from build123d import *

# Parameters (mm, degrees)
SKETCH1_W           = 80
SKETCH1_H           = 80
BOSS_EXTRUDE1_DEPTH = 14.5
FILLET1_R           = 2
FILLET2_R           = 4
SKETCH2_R           = 5.75
CUT_EXTRUDE1_DEPTH  = 2
SKETCH3_R           = 1.5
CUT_EXTRUDE2_DEPTH  = 12
SKETCH6_R           = 6
CUT_EXTRUDE3_DEPTH  = 2


with BuildPart() as part:
    # Sketch1 → Boss-Extrude1 (new, symmetric)
    with BuildSketch(Plane.XY):
        Rectangle(SKETCH1_W, SKETCH1_H)
    extrude(amount=BOSS_EXTRUDE1_DEPTH, both=True)

    # Fillet1
    fillet1_edges = [part.edges().sort_by_distance(p)[0] for p in [
        (-40, 0, 14.5),
        (0, -40, 14.5),
        (40, 0, 14.5),
        (0, 40, 14.5),
    ]]
    fillet(fillet1_edges, radius=FILLET1_R)

    # Fillet2
    # the kernel refuses this fillet: 4 mm, written as the material it takes off along each edge
    with BuildSketch(Plane(origin=(-36, -36, 14.5), x_dir=(-1, 0, 0), z_dir=(0, 1, 0))) as fillet2_piece_1:
        with BuildLine():
            CenterArc((2, -2), 2, 0, 90)
            Line((4, -2), (4, 0))
            Line((4, 0), (2, 0))
        make_face()
    revolve(axis=Axis((-36, -36, 14.5), (0, 0, 1)), revolution_arc=90, mode=Mode.SUBTRACT)
    with BuildSketch(Plane(origin=(-36, 36, 14.5), x_dir=(0, 1, 0), z_dir=(1, 0, 0))) as fillet2_piece_2:
        with BuildLine():
            CenterArc((2, -2), 2, 0, 90)
            Line((4, -2), (4, 0))
            Line((4, 0), (2, 0))
        make_face()
    revolve(axis=Axis((-36, 36, 14.5), (0, 0, 1)), revolution_arc=90, mode=Mode.SUBTRACT)
    with BuildSketch(Plane(origin=(36, -36, 14.5), x_dir=(0, -1, 0), z_dir=(-1, 0, 0))) as fillet2_piece_3:
        with BuildLine():
            CenterArc((2, -2), 2, 0, 90)
            Line((4, -2), (4, 0))
            Line((4, 0), (2, 0))
        make_face()
    revolve(axis=Axis((36, -36, 14.5), (0, 0, 1)), revolution_arc=90, mode=Mode.SUBTRACT)
    with BuildSketch(Plane(origin=(36, 36, 14.5), x_dir=(1, 0, 0), z_dir=(0, -1, 0))) as fillet2_piece_4:
        with BuildLine():
            CenterArc((2, -2), 2, 0, 90)
            Line((4, -2), (4, 0))
            Line((4, 0), (2, 0))
        make_face()
    revolve(axis=Axis((36, 36, 14.5), (0, 0, 1)), revolution_arc=90, mode=Mode.SUBTRACT)
    with BuildSketch(Plane(origin=(40, 40, 14.5), x_dir=(-1, 0, 0), z_dir=(0, 0, -1)), Plane(origin=(40, -40, 14.5), x_dir=(0, 1, 0), z_dir=(0, 0, -1)), Plane(origin=(-40, -40, -24.5), x_dir=(0, 1, 0), z_dir=(0, 0, 1)), Plane(origin=(-40, 40, -24.5), x_dir=(1, 0, 0), z_dir=(0, 0, 1))) as fillet2_piece_5:
        with BuildLine():
            CenterArc((FILLET2_R, -FILLET2_R), FILLET2_R, 90, 90)
            Line((0, -FILLET2_R), (0, 0))
            Line((0, 0), (FILLET2_R, 0))
        make_face()
    extrude(amount=39, mode=Mode.SUBTRACT)

    # Sketch2 → Cut-Extrude1 (cut)
    with BuildSketch(Plane.XY.offset(14.5)):
        with Locations((-27.6, 30.4)):
            Circle(SKETCH2_R)
        with Locations((-11.8, 30.4)):
            Circle(SKETCH2_R)
        with Locations((7.5, 30.4)):
            Circle(SKETCH2_R)
        with Locations((23.3, 30.4)):
            Circle(SKETCH2_R)
    extrude(amount=-CUT_EXTRUDE1_DEPTH, mode=Mode.SUBTRACT)

    # Sketch3 → Cut-Extrude2 (cut)
    with BuildSketch(Plane.XY.offset(14.5)):
        with Locations((-33.45, 21.95)):
            Circle(SKETCH3_R)
        with Locations((33.55, 21.95)):
            Circle(SKETCH3_R)
        with Locations((-33.45, -33.05)):
            Circle(SKETCH3_R)
        with Locations((33.55, -33.05)):
            Circle(SKETCH3_R)
    extrude(amount=-CUT_EXTRUDE2_DEPTH, mode=Mode.SUBTRACT)

    # Sketch6 → Cut-Extrude3 (cut)
    with BuildSketch(Plane.XY.offset(14.5)):
        with Locations((28.6, -16.4)):
            Circle(SKETCH6_R)
    extrude(amount=-CUT_EXTRUDE3_DEPTH, mode=Mode.SUBTRACT)


solid = part.part
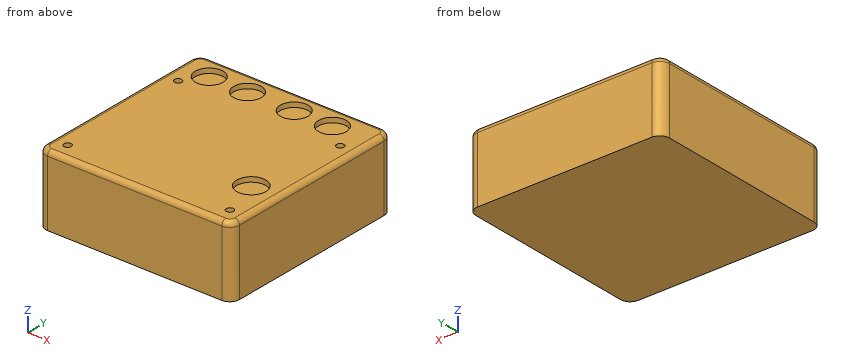
Geometry: final body of the model. Coordinates: model frame, mm. Give positions to 0.01 mm unless a question says otherwise; leave off trailing zeros. Write each loop counter-clockwise with the first axis right and the second up, starting at its lowest first coordinate (ties: lowest second). Pieces come first, ordered by that corner, then holes.
(1) Cut plane A-A, the plane y = 21.95. Return loops of the section in (x, z), then the cut area to 3 significant figures.
(2) Cut plane B-B, the plane y = 34.5. Return loops of the section in (x, z), then the cut area to 3 significant figures.
(3) First-contact query: P1, Ø7, axis at x = 7.5, y = 30.4, coming from the +Z side; P2, Ø1.8, axis at x = -33.45, y = -33.05, coming from the +Z side. Flat tips, straight axial feed; report the tip coordinate or a pass-through.
(4) Ray query, line 1 (Y direction, x = -33.45, z = 9); line 2 (Y direction, x = -27.6, z = 13.35); line 3 (Z direction, x = 9, y = 33). Return the intervals inside material, ascending.
Values follow:
1. outline: (-40, -14.5) - (40, -14.5) - (40, 12.5) arc R2 ccw to (38, 14.5) - (35.05, 14.5) - (35.05, 2.5) - (32.05, 2.5) - (32.05, 14.5) - (-31.95, 14.5) - (-31.95, 2.5) - (-34.95, 2.5) - (-34.95, 14.5) - (-38, 14.5) arc R2 ccw to (-40, 12.5) - close
1. area: 2,250 mm2
2. outline: (-40, -14.5) - (40, -14.5) - (40, 12.5) arc R2 ccw to (38, 14.5) - (27.33, 14.5) - (27.33, 12.5) - (19.27, 12.5) - (19.27, 14.5) - (11.53, 14.5) - (11.53, 12.5) - (3.47, 12.5) - (3.47, 14.5) - (-7.77, 14.5) - (-7.77, 12.5) - (-15.83, 12.5) - (-15.83, 14.5) - (-23.57, 14.5) - (-23.57, 12.5) - (-31.63, 12.5) - (-31.63, 14.5) - (-38, 14.5) arc R2 ccw to (-40, 12.5) - close
2. area: 2,250 mm2
3. P1: stops at z = 12.5
3. P2: stops at z = 2.5
4. line 1: y = -40 to -34.55, -31.55 to 20.45, 23.45 to 40
4. line 2: y = -39.81 to 24.65, 36.15 to 39.81
4. line 3: z = -14.5 to 12.5
